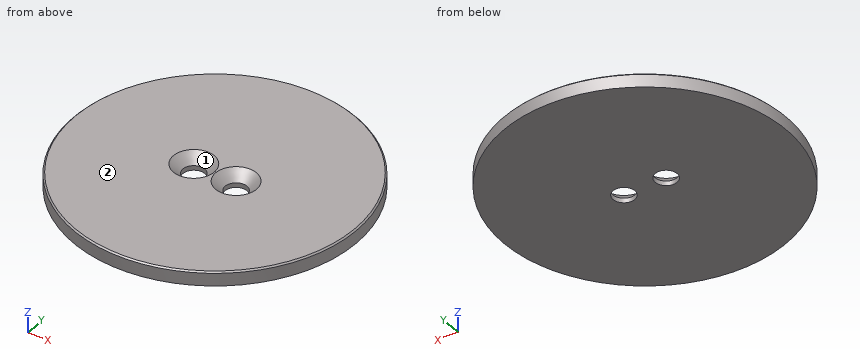
from build123d import *

# Parameters (mm, degrees)
SKETCH_1_R                   = 20
EXTRUDE_1_DEPTH              = 2
SKETCH_2_R                   = 1.55
CUT_EXTRUDE_1_DEPTH          = 2
HOLE_WIZARD_M3_1_D           = 3.1
HOLE_WIZARD_M3_1_DEPTH       = 10
HOLE_WIZARD_M3_1_CSINK_D     = 5.8
HOLE_WIZARD_M3_1_CSINK_ANGLE = 90
CHAMFER_1_SIZE               = 0.2


with BuildPart() as part:
    # 草图1 → 凸台-拉伸1 (new body)
    with BuildSketch(Plane.XY):
        Circle(SKETCH_1_R)
    extrude(amount=EXTRUDE_1_DEPTH)

    # 草图2 → 切除-拉伸1 (cut)
    with BuildSketch(Plane.XY.offset(2)):
        with Locations((-3, 0)):
            Circle(SKETCH_2_R)
        with Locations((3, 0)):
            Circle(SKETCH_2_R)
    extrude(amount=-CUT_EXTRUDE_1_DEPTH, mode=Mode.SUBTRACT)

    # M3 六角凹锥坑螺钉的锥形沉头孔1
    with Locations(Plane(origin=(-3, 0, 2), x_dir=(1, 0, 0), z_dir=(0, 0, 1))):
        with Locations((0, 0), (6, 0)):
            CounterSinkHole(HOLE_WIZARD_M3_1_D / 2, HOLE_WIZARD_M3_1_CSINK_D / 2, depth=HOLE_WIZARD_M3_1_DEPTH, counter_sink_angle=HOLE_WIZARD_M3_1_CSINK_ANGLE)

    # 倒角1
    chamfer_1_edges = [part.edges().sort_by_distance(p)[0] for p in [
        (-20, 0, 2),
    ]]
    chamfer(chamfer_1_edges, length=CHAMFER_1_SIZE)


solid = part.part
Design review of the part built by this model. Coordinates are the model's own, in mm. Face numbers are marked on the shaded views. Round coordinates to 2 decimals unless told otherwise and drop trailing zeros. Write each loop counter-clockwise with the first axis right and the second up, starting at its lowest first coordinate (ties: lowest second). Pieces come first, ordered by that corner, then holes. Notation, with made-up numbers: (49.25, 33.5) -> (63.25, 33.5) arc R20 cw to (63.25, 47.5) -> close; hole circle Ø11 at (20.5, -9). An arc over 180 degrees is marked (long way). One line per item, written item: value. Start each with the question number.
Q1. The part is to be moulded in two halves that separate along X. For the marked faces 1 and 2, say which applies: pulls with the +X half, pulls with the -X half, needs draft (parallel to the pull), parting line crosses it, or undercut.
Q2. To check wall thickness, follow probe 1 along Y at (x, z) = (-3, 0.55); probe 2 along Y at (x, z) = (-5, 1.65); probe 3 along X at (y, z) = (3, 1.35). State the ranges of each line that lie inside material, in increasing order.
Q3. Add section A-A (y = 0). Give the boundary of the cut face in (x, z), then the cut area to 3 significant figures.
Q4. Add section B-B (z = 1). Give the boundary of the cut face in (x, y), then the cut area to 3 significant figures.
Response:
1. face 1: undercut
1. face 2: needs draft
2. probe 1: y = -19.77 to -1.55, 1.55 to 19.77
2. probe 2: y = -19.36 to -1.58, 1.58 to 19.36
2. probe 3: x = -19.77 to 19.77
3. outline: (-20, 0) -> (-4.55, 0) -> (-4.55, 0.65) -> (-5.9, 2) -> (-19.8, 2) -> (-20, 1.8) -> close; (-1.45, 0) -> (1.45, 0) -> (1.45, 0.65) -> (0.1, 2) -> (-0.1, 2) -> (-1.45, 0.65) -> close; (4.55, 0) -> (20, 0) -> (20, 1.8) -> (19.8, 2) -> (5.9, 2) -> (4.55, 0.65) -> close
3. area: 63.9 mm^2
4. outline: circle Ø40 at (0, 0); hole circle Ø3.8 at (-3, 0); hole circle Ø3.8 at (3, 0)
4. area: 1,230 mm^2
